Geometry: see drawing. Coordinates: mm, zero at the bounding-box minimum. Round coordinates to 2 decimals unless told otherwise and drop trailing zeros. Loops run counter-clockwise (first coordinate to the right, second up) from the corner with the lowest first, then second, coordinate; pieces in that order, holes last. Notation, with made-up numbers: (0.25, 64.25) - (16.25, 64.25) arc R19 ccw to (16.25, 97.25) - close; hole circle Ø3 at (32, -1). An arc over 180 degrees is marked (long way). One line per question, with ' | ' between items. Start each with the question number.
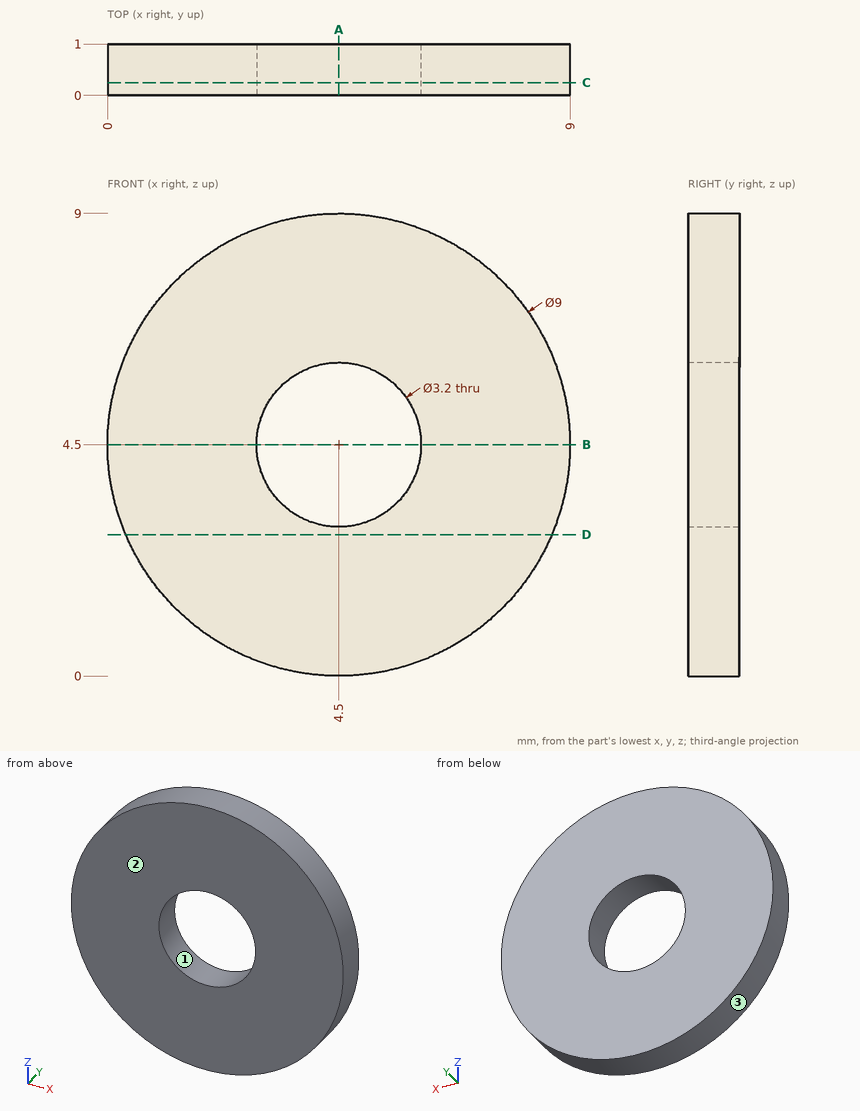
(1) Section A-A, the plane x = 4.5. Output: boundary loops of the cut face in (y, z).
(2) Pull-direction query (Z, two-part tool) for the marked faces 1, 2 and 3; classes: released by +Z, released by -Z, zero draft, split by the parting line, or undercut.
(3) Line query: line 1 along Z through (x, y) = (4.5, 0.6); line 2 along X through (y, z) = (0.85, 5); line 3 along X through (y, z) = (0.9, 4.25). Output: solid intervals per line, ascending. Write a range as from..to.
(4) Section B-B, the plane z = 4.5. Output: boundary loops of the cut face in (x, y).
(5) Section D-D, the plane z = 2.75. Output: boundary loops of the cut face in (x, y), plus the area to 3 significant figures.
(6) Section C-C, the plane y = 0.25. Output: boundary loops of the cut face in (x, z).
Derived:
1) outline: (0, 0) - (1, 0) - (1, 2.9) - (0, 2.9) - close; (0, 6.1) - (1, 6.1) - (1, 9) - (0, 9) - close
2) face 1: undercut | face 2: zero draft | face 3: split by the parting line
3) line 1: z = 0..2.9, 6.1..9 | line 2: x = 0.03..2.98, 6.02..8.97 | line 3: x = 0.01..2.92, 6.08..8.99
4) outline: (0, 0) - (2.9, 0) - (2.9, 1) - (0, 1) - close; (6.1, 0) - (9, 0) - (9, 1) - (6.1, 1) - close
5) outline: (0.35, 0) - (8.65, 0) - (8.65, 1) - (0.35, 1) - close | area: 8.29 mm²
6) outline: circle Ø9 at (4.5, 4.5); hole circle Ø3.2 at (4.5, 4.5)
